from build123d import *

# Parameters (mm, degrees)
ESQUISSE1_W             = 100
ESQUISSE1_H             = 100
BOSS_EXTRU_1_DEPTH      = 10
ESQUISSE3_R             = 4
ESQUISSE3_R_2           = 1.25
ENL_V_MAT_EXTRU_2_DEPTH = 200.246053595


with BuildPart() as part:
    # Esquisse1 → Boss.-Extru.1 (new body)
    with BuildSketch(Plane.XY):
        with BuildLine():
            ThreePointArc((-100.822483701, 122.822483701), (-134.852813742, 134.852813742), (-122.822483701, 100.822483701))
            Line((-122.822483701, 100.822483701), (-131.710678119, 109.710678119))
            Line((-131.710678119, 109.710678119), (-109.710678119, 131.710678119))
            Line((-109.710678119, 131.710678119), (-100.822483701, 122.822483701))
        make_face()
        with BuildLine():
            Line((-131.710678119, 109.710678119), (-122.822483701, 100.822483701))
            ThreePointArc((-122.822483701, 100.822483701), (-107.336002639, 105.840639254), (-100.710678119, 120.710678119))
            ThreePointArc((-100.710678119, 120.710678119), (-100.738649074, 121.768059709), (-100.822483701, 122.822483701))
            Line((-100.822483701, 122.822483701), (-109.710678119, 131.710678119))
            Line((-109.710678119, 131.710678119), (-131.710678119, 109.710678119))
        make_face()
        with BuildLine():
            Line((-122.822483701, 100.822483701), (-50, 28))
            Line((-50, 28), (-50, 50))
            Line((-50, 50), (-28, 50))
            Line((-28, 50), (-100.822483701, 122.822483701))
            ThreePointArc((-100.822483701, 122.822483701), (-100.738649074, 121.768059709), (-100.710678119, 120.710678119))
            ThreePointArc((-100.710678119, 120.710678119), (-107.336002639, 105.840639254), (-122.822483701, 100.822483701))
        make_face()
        with BuildLine():
            Line((100.822483701, 122.822483701), (28, 50))
            Line((28, 50), (50, 50))
            Line((50, 50), (50, 28))
            Line((50, 28), (122.822483701, 100.822483701))
            ThreePointArc((122.822483701, 100.822483701), (106.568542495, 106.568542495), (100.822483701, 122.822483701))
        make_face()
        with BuildLine():
            ThreePointArc((140.710678119, 120.710678119), (121.768059709, 140.682707164), (100.822483701, 122.822483701))
            Line((100.822483701, 122.822483701), (109.710678119, 131.710678119))
            Line((109.710678119, 131.710678119), (131.710678119, 109.710678119))
            Line((131.710678119, 109.710678119), (122.822483701, 100.822483701))
            ThreePointArc((122.822483701, 100.822483701), (135.580716983, 107.336002639), (140.710678119, 120.710678119))
        make_face()
        with BuildLine():
            Line((109.710678119, 131.710678119), (100.822483701, 122.822483701))
            ThreePointArc((100.822483701, 122.822483701), (106.568542495, 106.568542495), (122.822483701, 100.822483701))
            Line((122.822483701, 100.822483701), (131.710678119, 109.710678119))
            Line((131.710678119, 109.710678119), (109.710678119, 131.710678119))
        make_face()
        Rectangle(ESQUISSE1_W, ESQUISSE1_H)
        with BuildLine():
            ThreePointArc((122.822483701, -100.822483701), (106.568542495, -106.568542495), (100.822483701, -122.822483701))
            Line((100.822483701, -122.822483701), (109.710678119, -131.710678119))
            Line((109.710678119, -131.710678119), (131.710678119, -109.710678119))
            Line((131.710678119, -109.710678119), (122.822483701, -100.822483701))
        make_face()
        with BuildLine():
            Line((109.710678119, -131.710678119), (100.822483701, -122.822483701))
            ThreePointArc((100.822483701, -122.822483701), (121.768059709, -140.682707164), (140.710678119, -120.710678119))
            ThreePointArc((140.710678119, -120.710678119), (135.580716983, -107.336002639), (122.822483701, -100.822483701))
            Line((122.822483701, -100.822483701), (131.710678119, -109.710678119))
            Line((131.710678119, -109.710678119), (109.710678119, -131.710678119))
        make_face()
        with BuildLine():
            Line((50, -50), (28, -50))
            Line((28, -50), (100.822483701, -122.822483701))
            ThreePointArc((100.822483701, -122.822483701), (106.568542495, -106.568542495), (122.822483701, -100.822483701))
            Line((122.822483701, -100.822483701), (50, -28))
            Line((50, -28), (50, -50))
        make_face()
        with BuildLine():
            ThreePointArc((-100.710678119, -120.710678119), (-107.336002639, -105.840639254), (-122.822483701, -100.822483701))
            Line((-122.822483701, -100.822483701), (-131.710678119, -109.710678119))
            Line((-131.710678119, -109.710678119), (-109.710678119, -131.710678119))
            Line((-109.710678119, -131.710678119), (-100.822483701, -122.822483701))
            ThreePointArc((-100.822483701, -122.822483701), (-100.738649074, -121.768059709), (-100.710678119, -120.710678119))
        make_face()
        with BuildLine():
            Line((-131.710678119, -109.710678119), (-122.822483701, -100.822483701))
            ThreePointArc((-122.822483701, -100.822483701), (-134.852813742, -134.852813742), (-100.822483701, -122.822483701))
            Line((-100.822483701, -122.822483701), (-109.710678119, -131.710678119))
            Line((-109.710678119, -131.710678119), (-131.710678119, -109.710678119))
        make_face()
        with BuildLine():
            Line((-50, -50), (-50, -28))
            Line((-50, -28), (-122.822483701, -100.822483701))
            ThreePointArc((-122.822483701, -100.822483701), (-107.336002639, -105.840639254), (-100.710678119, -120.710678119))
            ThreePointArc((-100.710678119, -120.710678119), (-100.738649074, -121.768059709), (-100.822483701, -122.822483701))
            Line((-100.822483701, -122.822483701), (-28, -50))
            Line((-28, -50), (-50, -50))
        make_face()
    extrude(amount=BOSS_EXTRU_1_DEPTH)

    # Esquisse3 → Enlèv. mat.-Extru.2 (cut, through all)
    with BuildSketch(Plane(origin=(0, 0, 0), x_dir=(-1, 0, 0), z_dir=(0, 0, -1))):
        with Locations((-78.284271247, 78.284271247)):
            Circle(ESQUISSE3_R)
        with Locations((-24.748737342, 24.748737342)):
            Circle(ESQUISSE3_R)
        with Locations((78.284271247, 78.284271247)):
            Circle(ESQUISSE3_R)
        with Locations((24.748737342, 24.748737342)):
            Circle(ESQUISSE3_R)
        with Locations((78.284271247, -78.284271247)):
            Circle(ESQUISSE3_R)
        with Locations((24.748737342, -24.748737342)):
            Circle(ESQUISSE3_R)
        with Locations((-78.284271247, -78.284271247)):
            Circle(ESQUISSE3_R)
        with Locations((-24.748737342, -24.748737342)):
            Circle(ESQUISSE3_R)
        with Locations((-37.92, 0)):
            Circle(ESQUISSE3_R_2)
        with Locations((0, 37.92)):
            Circle(ESQUISSE3_R_2)
        with Locations((37.92, 0)):
            Circle(ESQUISSE3_R_2)
        with Locations((0, -37.92)):
            Circle(ESQUISSE3_R_2)
    extrude(amount=-ENL_V_MAT_EXTRU_2_DEPTH, mode=Mode.SUBTRACT)


solid = part.part
CAD build for the part. Positions are in the model's coordinates, mm. A direction names the side the tool comes from. Give positions to 0.01 mm unless a question says otherwise; leave off trailing zeros. Write each loop counter-clockwise with the first axis right and the second up, starting at its lowest first coordinate (ties: lowest second). Pieces come first, ordered by that corner, then holes. Notation, with made-up numbers: (53, 5) -> (63, 5) arc R6 ccw to (63, 9) -> close; hole circle Ø3 at (-20, -9). An arc over 180 degrees is marked (long way). Return JSON: item names as keys, results as strings.
Item 1: Band-saw the part on B-B (y = 110.5). List the corners of the cut face in (x, z).
Answer below:
{"outline": "(-137.91, 0) -> (-88.5, 0) -> (-88.5, 10) -> (-137.91, 10) -> close; (88.5, 0) -> (137.91, 0) -> (137.91, 10) -> (88.5, 10) -> close"}
Item 2: Band-saw the part on C-C (z = 6.5). Give the number of separate pieces and of enclosed holes in the cut face, then the cut area to 3 significant figures.
Answer below:
{"separate pieces": "1", "enclosed holes": "12", "area": "25,800 mm2"}
Item 3: Drill centre lines: probe 1 along X at (y, z) = (27.5, 9.75); probe 2 along Y at (x, z) = (24, 5.75); probe 3 along Y at (x, z) = (-113.5, 8). Where is each one in solid material? Low to high.
Answer below:
{"probe 1": "x = -50 to -27.65, -21.85 to 21.85, 27.65 to 50", "probe 2": "y = -50 to -28.68, -20.82 to 20.82, 28.68 to 50", "probe 3": "y = -139.37 to -91.5, 91.5 to 139.37"}
Item 4: Two-plate mould, pull along X, no slides. Class faces 4 (the flat face through (-1, -10, 10)), 5 (the cylindrical face through (-134.4, 135.29, 4.93)), 6 (the flat face through (50, 0, 5)): +X half, -X half, draft (parallel to the pull), parting line (faces both ways), or undercut.
Answer below:
{"face 4": "draft", "face 5": "undercut", "face 6": "+X half"}
Item 5: Tool access for faces 1 (the flat face through (64, -86, 5)), 2 (the flat face through (86, 64, 5)), 3 (the flat face through (-50, 0, 5)): list every direction of +Z, -Z, +X, -X, +Y, -Y with a clear straight run to the whole face (end or side of a thin tool).
Answer below:
{"face 1": "+Z, -Z, -Y", "face 2": "+Z, -Z, +X", "face 3": "+Z, -Z, -X"}
Item 6: Band-saw the part on A-A (x = 70). List the corners of the cut face in (y, z).
Answer below:
{"outline": "(-92, 0) -> (-48, 0) -> (-48, 10) -> (-92, 10) -> close; (48, 0) -> (92, 0) -> (92, 10) -> (48, 10) -> close"}
Item 7: Drop flat-ended pins along their axis: pin 1 (3 mm diameter, centred on x = -65.5, z = 1, fed in from +Y); pin 2 (9 mm diameter, centred on x = 24.75, y = -24.75, fed in from +Z); pin 3 (6 mm diameter, centred on x = -43, z = 8, fed in from -Y); pin 4 (6 mm diameter, centred on x = 78.5, z = 6, fed in from +Y). Give the stop position or say it passes through.
Answer below:
{"pin 1": "stops at y = 89", "pin 2": "stops at z = 10", "pin 3": "stops at y = -68", "pin 4": "stops at y = 103.5"}
